from build123d import *

# Parameters (mm, degrees)
EXTRUDE_1_DEPTH     = 6
SKETCH_2_R          = 5.5
EXTRUDE_2_DEPTH     = 11.5
SKETCH_3_R          = 2
CUT_EXTRUDE_1_DEPTH = 17.5
FILLET_1_R          = 0.5
FILLET_2_R          = 0.5
FILLET_3_R          = 0.5


with BuildPart() as part:
    # 草图1 → 凸台-拉伸1 (new body)
    with BuildSketch(Plane.XY):
        Polygon((-6.352433325, 2.765246979), (-5.570990794, -4.118745146), (0.781442531, -6.883992125), (6.352433325, -2.765246979), (5.570990794, 4.118745146), (-0.781442531, 6.883992125), align=None)
    extrude(amount=EXTRUDE_1_DEPTH)

    # 草图2 → 凸台-拉伸2 (add)
    with BuildSketch(Plane.XY):
        Circle(SKETCH_2_R)
    extrude(amount=-EXTRUDE_2_DEPTH)

    # 草图3 → 切除-拉伸1 (cut)
    with BuildSketch(Plane(origin=(0, 0, -11.5), x_dir=(-1, 0, 0), z_dir=(0, 0, -1))):
        Circle(SKETCH_3_R)
    extrude(amount=-CUT_EXTRUDE_1_DEPTH, mode=Mode.SUBTRACT)

    # 圆角1
    fillet_1_edges = [part.edges().sort_by_distance(p)[0] for p in [
        (-5.5, 0, 0),
    ]]
    fillet(fillet_1_edges, radius=FILLET_1_R - 0.0001)  # a hair under: the kernel refuses the full size

    # 圆角2
    fillet_2_edges = [part.edges().sort_by_distance(p)[0] for p in [
        (-2.394774131, -5.501368635, 6),
        (3.566937928, -4.824619552, 6),
        (5.961712059, 0.676749083, 6),
        (-5.5, 0, -11.5),
        (2.394774131, 5.501368635, 6),
        (-3.566937928, 4.824619552, 6),
        (-5.961712059, -0.676749083, 6),
    ]]
    fillet(fillet_2_edges, radius=FILLET_2_R)

    # 圆角3
    fillet_3_edges = [part.edges().sort_by_distance(p)[0] for p in [
        (2, 0, -11.5),
        (2, 0, 6),
    ]]
    fillet(fillet_3_edges, radius=FILLET_3_R)


solid = part.part
Work out the finished part from the listing and answer in its coordinate system (mm). Round coordinates to 2 decimals unless told otherwise and drop trailing zeros. Write each loop counter-clockwise with the first axis right and the second up, starting at its lowest first coordinate (ties: lowest second). Pieces come first, ordered by that corner, then holes.
1) Straight lines are drawn through the part: line 1 (Y direction, x = 0, z = -5.75); line 2 (Y direction, x = -4, z = -4.5); line 3 (Y direction, x = 0, z = 1.75). For each, find the intervals that lie inside material, in ascending order.
2) Given pin 1 Ø1.5 at (x, z) = (-4.5, -1) entering from +Y; pin 2 Ø1 at (y, z) = (-2.5, -3) entering from -X; pin 3 Ø2 at (y, z) = (-2, -8) entering from -X, each flat-ended and moving along its own axis, determine where each tip first touches the part or whether it passes through.
3) A cutting plane is placed at A-A (z = 1.5). Give the vertices of the cut face in (x, y), plus the area to 3 significant figures.
4) The mould has two halves that part along Y. Classify faces 1 (the cylindrical face through (-5.815, -0.709, 5.85)), 2 (the cylindrical face through (0, -2, -3)), 3 (the cylindrical face through (-1.19, -5.37, -5.68)), 4 (the cylindrical face through (2.29, 5.39, 5.85)): pulls with the +Y half, pulls with the -Y half, needs draft (parallel to the pull), parting line crosses it, or undercut.
5) A cutting plane is placed at B-B (z = -8.75). Give the vertices of the cut face in (x, y).
Completed:
1. line 1: y = -5.5 to -2, 2 to 5.5
1. line 2: y = -3.77 to 3.77
1. line 3: y = -6.54 to -2, 2 to 6.54
2. pin 1: stops at y = 4.02
2. pin 2: stops at x = -5.12
2. pin 3: stops at x = -5.41
3. outline: (-6.35, 2.77) - (-5.57, -4.12) - (0.78, -6.88) - (6.35, -2.77) - (5.57, 4.12) - (-0.78, 6.88) - close; hole circle Ø4 at (0, 0)
3. area: 112 mm2
4. face 1: pulls with the -Y half
4. face 2: undercut
4. face 3: parting line crosses it
4. face 4: pulls with the +Y half
5. outline: circle Ø11 at (0, 0); hole circle Ø4 at (0, 0)
